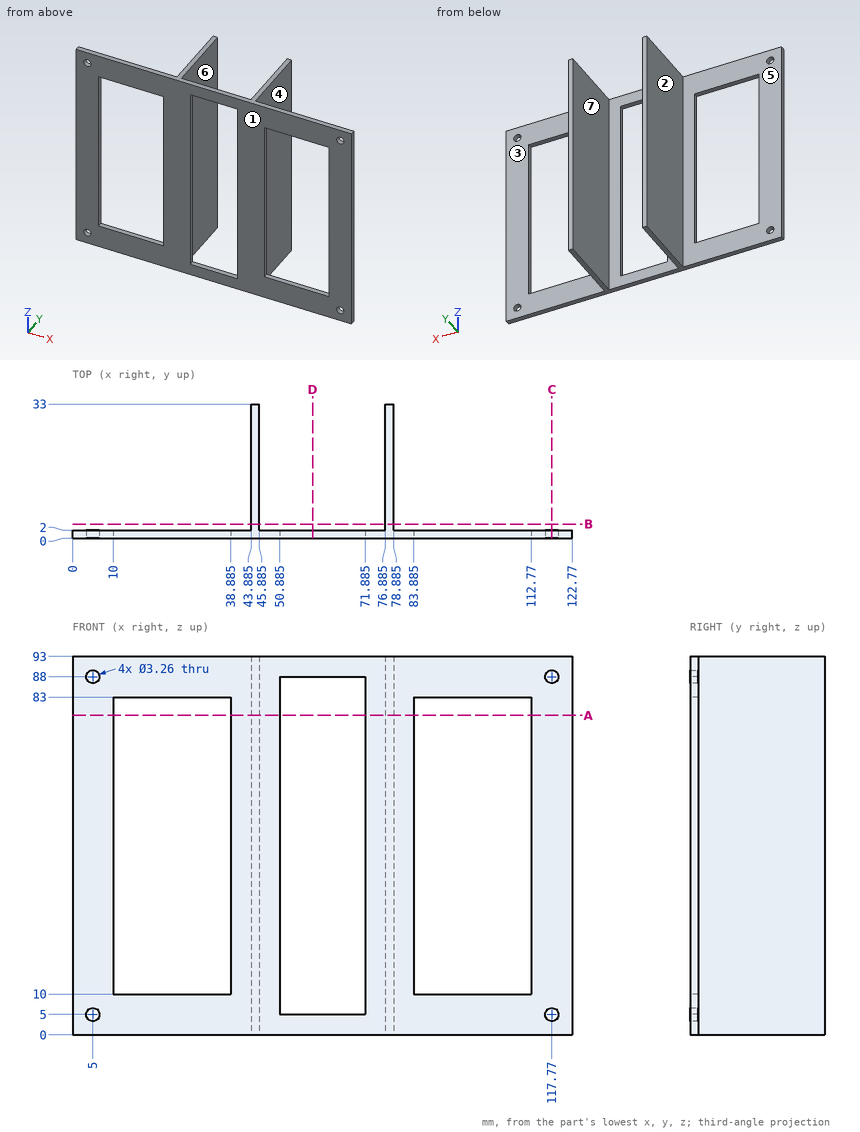
Input: dimensioned drawing with shaded views. Units: mm. Origin: part minimum x, y, z. A direction names the side the tool comes from. Round coordinates to 2 decimals unless told otherwise and drop trailing zeros. Loops run counter-clockwise (first coordinate to the right, second up) from the corner with the lowest first, then second, coordinate; pieces in that order, holes last. Notation, with made-up numbers: M -36.5,6 L -2.5,6 A13 cw -2.5,10 Z; hole C 13,84 d5. An arc over 180 degrees is marked long. Answer in a Markdown table with one row per item. Add a question column.
1. Set-up query: the marked faces 1, 2 and 3. Return all of +Z, -Z, +X, -X, +Y, -Y with unobstructed straight access to the full face (end or side cutting, diameter ignored); none if empty.
2. Section B-B (y = 3.5). Output: boundary loops of the cut face in (x, z) (3 decimals).
3. Section A-A (z = 78.5). Output: boundary loops of the cut face in (x, y) (3 decimals).
4. Section D-D (x = 59). Output: boundary loops of the cut face in (y, z).
5. Contact query for flat-ended pins moving along their axis: pin 1 (12 mm diameter, centred on y = 14.5, z = 74.5, fed in from -X) (3 decimals); pin 2 (2 mm diameter, centred on y = 15.5, z = 76, fed in from +X) (3 decimals); pin 3 (3 mm diameter, centred on x = 50, z = 69, fed in from +Y). Output: stop coordinate, or through.
6. Mould query, pull axis X, two halves, no side actions, for the marked faces 4, 5, 6 and 7. Classes: released by +X, released by -X, zero draft, split by the parting line, or undercut.
7. Ray query, probe 1 along X at (y, z) = (1, 72) (3 decimals); probe 2 along X at (y, z) = (8, 5.5) (3 decimals); probe 3 along Y at (x, z) = (115, 39). Return the intervals inside material, ascending.
8. Section C-C (x = 117.77). Output: boundary loops of the cut face in (y, z).
Values follow:
| question | item | result |
|---|---|---|
| 1 | face 1 | +Z, -Z, +X, -X, -Y |
| 1 | face 2 | +Z, -Z, -X, +Y |
| 1 | face 3 | +Z, -Z, +X, +Y |
| 2 | outline | M 43.885,0 L 45.885,0 L 45.885,93 L 43.885,93 Z; M 76.885,0 L 78.885,0 L 78.885,93 L 76.885,93 Z |
| 3 | outline | M 0,0 L 10,0 L 10,2 L 0,2 Z; M 38.885,0 L 50.885,0 L 50.885,2 L 45.885,2 L 45.885,33 L 43.885,33 L 43.885,2 L 38.885,2 Z; M 71.885,0 L 83.885,0 L 83.885,2 L 78.885,2 L 78.885,33 L 76.885,33 L 76.885,2 L 71.885,2 Z; M 112.77,0 L 122.77,0 L 122.77,2 L 112.77,2 Z |
| 4 | outline | M 0,0 L 2,0 L 2,5 L 0,5 Z; M 0,88 L 2,88 L 2,93 L 0,93 Z |
| 5 | pin 1 | x = 43.885 |
| 5 | pin 2 | x = 78.885 |
| 5 | pin 3 | y = 2 |
| 6 | face 4 | released by +X |
| 6 | face 5 | zero draft |
| 6 | face 6 | undercut |
| 6 | face 7 | undercut |
| 7 | probe 1 | 0 to 10, 38.885 to 50.885, 71.885 to 83.885, 112.77 to 122.77 |
| 7 | probe 2 | 43.885 to 45.885, 76.885 to 78.885 |
| 7 | probe 3 | 0 to 2 |
| 8 | outline | M 0,0 L 2,0 L 2,3.37 L 0,3.37 Z; M 0,6.63 L 2,6.63 L 2,86.37 L 0,86.37 Z; M 0,89.63 L 2,89.63 L 2,93 L 0,93 Z |
